Geometry: final body of the model. Coordinates: model frame, mm. A direction names the side the tool comes from. Round coordinates to 2 decimals unless told otherwise and drop trailing zeros. Order: outer loops, then holes, each group sorted by start corner. A loop starts at its lowest first (then second) coordinate and runs counter-clockwise, first axis right, second up. Notation, with made-up numbers: M -18,63 L 14,63 A16 cw 14,70 Z; hole C 6,-29 d10. An arc over 180 degrees is marked long. Return JSON: item names as keys, results as strings. Group by question number.
Q1. Cut plane C-C on x = -1.5. Output: boundary loops of the cut face in (y, z), and give its area (3 significant figures).
Q2. Mould query, pull axis Y, two halves, no side actions, for faces 1 (the face through (-3.5, 0, 4)), 2 (the face through (2.5, 0, 4)). Classes: released by +Y, released by -Y, zero draft, split by the parting line, or undercut.
Q3. Cut plane A-A on y = 6.75. Output: boundary loops of the cut face in (x, z), and give its area (3 significant figures).
Q4. Access query for faces 3 (the face through (-2.5, 0, 4)), 4 (the face through (-3, 2, 0)). Directions: +Z, -Z, +X, -X, +Y, -Y. A direction counts if a zero-diameter tool reaches every point of the face in a straight line with its end or side. Return the directions, or none.
Q5. Cut plane D-D on x = 0.75. Output: boundary loops of the cut face in (y, z).
Q6. Ray query, probe 1 along X at (y, z) = (1.5, 3.5); probe 2 along Y at (x, z) = (-2.25, 1.5); probe 3 along Y at (x, z) = (-3, 4.75). Return the intervals inside material, ascending.
Q7. Contact query for a flat-ended pin moving along its axis: pin 1 (1.5 mm diameter, centred on x = -0.5, y = -7.5, fed in from +Z). Output: stop coordinate, or through.
```python
from build123d import *

# Parameters (mm, degrees)
F1_DEPTH = 8
F2_R     = 0.5
F3_SIZE  = 0.49999


# Not quite as in the source:
# - a fillet or chamfer is up to 0.001 mm smaller than in the source, because OpenCascade refuses the exact size


with BuildPart() as f1:
    # F0 (on Top) → F1 (new body)
    with BuildSketch(Plane.XY):
        with BuildLine():
            Line((-2.5, -12.75), (-2.5, 12.75))
            ThreePointArc((-2.5, 12.75), (-1.767766953, 14.517766953), (0, 15.25))
            ThreePointArc((0, 15.25), (1.767766953, 14.517766953), (2.5, 12.75))
            Line((2.5, 12.75), (2.5, -12.75))
            Line((2.5, -12.75), (2, -12.75))
            Line((2, -12.75), (2, -13.75))
            Line((2, -13.75), (3.5, -13.75))
            Line((3.5, -13.75), (3.5, 12.75))
            ThreePointArc((3.5, 12.75), (2.4748737342, 15.2248737342), (0, 16.25))
            ThreePointArc((0, 16.25), (-2.4748737342, 15.2248737342), (-3.5, 12.75))
            Line((-3.5, 12.75), (-3.5, -13.75))
            Line((-3.5, -13.75), (-2, -13.75))
            Line((-2, -13.75), (-2, -12.75))
            Line((-2, -12.75), (-2.5, -12.75))
        make_face()
    extrude(amount=F1_DEPTH)

    # F2
    f2_edges = [f1.edges().sort_by_distance(p)[0] for p in [
        (-3.5, -13.75, 4),
        (3.5, -13.75, 4),
    ]]
    fillet(f2_edges, radius=F2_R)

    # F3 (size 0.5 in the source; OpenCascade refuses exactly that, so slightly less here)
    f3_edges = [f1.edges().sort_by_distance(p)[0] for p in [
        (-2, -13.75, 4),
        (-2, -12.75, 4),
        (2, -13.75, 4),
        (2, -12.75, 4),
    ]]
    chamfer(f3_edges, length=F3_SIZE)


solid = f1.part
```
Result sheet:
{
 "1": {"outline": "M 14.75,0 L 15.91,0 L 15.91,8 L 14.75,8 Z", "area": "9.30 mm²"},
 "2": {"face 1": "zero draft", "face 2": "undercut"},
 "3": {"outline": "M -3.5,0 L -2.5,0 L -2.5,8 L -3.5,8 Z; M 2.5,0 L 3.5,0 L 3.5,8 L 2.5,8 Z", "area": "16.0 mm²"},
 "4": {"face 3": "+Z, -Z", "face 4": "-Z, +X, -X, +Y, -Y"},
 "5": {"outline": "M 15.13,0 L 16.17,0 L 16.17,8 L 15.13,8 Z"},
 "6": {"probe 1": "x = -3.5 to -2.5, 2.5 to 3.5", "probe 2": "y = -13.5 to -13, 13.84 to 15.43", "probe 3": "y = -13.75 to 14.55"},
 "7": {"pin 1": "passes through"}
}
